```python
from build123d import *

# Parameters (mm, degrees)
SKETCH1_W       = 39
SKETCH1_H       = 39
EXTRUDE1_DEPTH  = 150
SKETCH2_W       = 36
SKETCH2_H       = 36
EXTRUDE2_DEPTH  = 112
SKETCH3_W       = 4.5
SKETCH3_H       = 120
EXTRUDE3_DEPTH  = 158.167148993
SKETCH8_W       = 36
SKETCH8_H       = 33
EXTRUDE6_DEPTH  = 2
FILLET1_R       = 1.5
SKETCH11_W      = 23.29
SKETCH11_H      = 15
EXTRUDE8_DEPTH  = 158.167148993
EXTRUDE9_DEPTH  = 1.5
SKETCH14_R      = 1.45
EXTRUDE11_DEPTH = 1.5
SKETCH15_R      = 10.365721684
EXTRUDE12_DEPTH = 158.167148993
SKETCH17_W      = 4.5
SKETCH17_H      = 1
EXTRUDE14_DEPTH = 158.167148993
SKETCH18_W      = 34.5
SKETCH18_H      = 34.16
EXTRUDE15_DEPTH = 158.167148993
SKETCH19_W      = 5
SKETCH19_H      = 10.5
EXTRUDE16_DEPTH = 10
SKETCH20_W      = 5
SKETCH20_H      = 10.5
EXTRUDE17_DEPTH = 10
SKETCH21_R      = 1.6
EXTRUDE18_DEPTH = 10
SKETCH22_R      = 1.6
EXTRUDE19_DEPTH = 10
EXTRUDE20_DEPTH = 5
SKETCH25_R      = 10
EXTRUDE21_DEPTH = 5
EXTRUDE23_DEPTH = 4
FILLET2_R       = 10
FILLET3_R       = 2


with BuildPart() as part:
    # Sketch1 → Extrude1 (new body)
    with BuildSketch(Plane(origin=(0, 0, 0), x_dir=(1, 0, 0), z_dir=(0, 1, 0))):
        with Locations((-11.707942094, -6.586638776)):
            Rectangle(SKETCH1_W, SKETCH1_H)
    extrude(amount=EXTRUDE1_DEPTH)

    # Sketch2 → Extrude2 (cut)
    with BuildSketch(Plane(origin=(0, 150, 0), x_dir=(1, 0, 0), z_dir=(0, 1, 0))):
        with Locations((-11.707942094, -6.586638776)):
            Rectangle(SKETCH2_W, SKETCH2_H)
    extrude(amount=-EXTRUDE2_DEPTH, mode=Mode.SUBTRACT)

    # Sketch3 → Extrude3 (cut, through all)
    with BuildSketch(Plane.ZY.offset(31.207942094)):
        with Locations((23.836638776, 60)):
            Rectangle(SKETCH3_W, SKETCH3_H)
    extrude(amount=-EXTRUDE3_DEPTH, mode=Mode.SUBTRACT)

    # Sketch8 → Extrude6 (cut)
    with BuildSketch(Plane(origin=(0, 38, 0), x_dir=(1, 0, 0), z_dir=(0, 1, 0))):
        with Locations((-11.707942094, -5.086638776)):
            Rectangle(SKETCH8_W, SKETCH8_H)
    extrude(amount=-EXTRUDE6_DEPTH, mode=Mode.SUBTRACT)

    # Fillet1
    fillet1_edges = [part.edges().sort_by_distance(p)[0] for p in [
        (-29.707942094, 93, -11.413361224),
        (6.292057906, 93, -11.413361224),
        (6.292057906, 135, 24.586638776),
        (-29.707942094, 135, 24.586638776),
        (6.292057906, 36, 5.086638776),
        (-29.707942094, 36, 5.086638776),
        (-11.707942094, 36, -11.413361224),
    ]]
    fillet(fillet1_edges, radius=FILLET1_R)

    # Sketch11 → Extrude8 (cut, through all)
    with BuildSketch(Plane.ZY.offset(31.207942094)):
        with BuildLine():
            Line((-3.255937041, 62.910708566), (-3.255937041, 92.357092416))
            ThreePointArc((-3.255937041, 92.357092416), (3.739612713, 99.352642171), (10.735162468, 92.357092416))
            Line((10.735162468, 92.357092416), (10.735162468, 62.910708566))
            ThreePointArc((10.735162468, 62.910708566), (3.739612713, 55.915158812), (-3.255937041, 62.910708566))
        make_face()
        with Locations((6.591638776, 142.5)):
            Rectangle(SKETCH11_W, SKETCH11_H)
    extrude(amount=-EXTRUDE8_DEPTH, mode=Mode.SUBTRACT)

    # Sketch12 → Extrude9 (cut)
    with BuildSketch(Plane(origin=(0, 0, -12.913361224), x_dir=(-1, 0, 0), z_dir=(0, 0, -1))):
        with BuildLine():
            Line((5.065703237, 62.27828297), (5.065703237, 91.808021534))
            ThreePointArc((5.065703237, 91.808021534), (11.707942094, 98.450260391), (18.350180951, 91.808021534))
            Line((18.350180951, 91.808021534), (18.350180951, 62.27828297))
            ThreePointArc((18.350180951, 62.27828297), (11.707942094, 55.636044113), (5.065703237, 62.27828297))
        make_face()
        with BuildLine():
            Line((6.527758749, 115.3801061), (6.527758749, 136.80161472))
            ThreePointArc((6.527758749, 136.80161472), (11.707942094, 141.981798065), (16.888125439, 136.80161472))
            Line((16.888125439, 136.80161472), (16.888125439, 115.3801061))
            ThreePointArc((16.888125439, 115.3801061), (11.707942094, 110.199922755), (6.527758749, 115.3801061))
        make_face()
    extrude(amount=-EXTRUDE9_DEPTH, mode=Mode.SUBTRACT)

    # Sketch14 → Extrude11 (cut)
    with BuildSketch(Plane.XY.offset(26.086638776)):
        with Locations((-5.707942094, 138.35)):
            Circle(SKETCH14_R)
        with Locations((-17.707942094, 138.35)):
            Circle(SKETCH14_R)
    extrude(amount=-EXTRUDE11_DEPTH, mode=Mode.SUBTRACT)

    # Sketch15 → Extrude12 (cut, through all)
    with BuildSketch(Plane.ZY.offset(31.207942094)):
        with Locations((3.739612713, 119.241924714)):
            Circle(SKETCH15_R)
    extrude(amount=-EXTRUDE12_DEPTH, mode=Mode.SUBTRACT)

    # Sketch17 → Extrude14 (cut, through all)
    with BuildSketch(Plane.ZY.offset(31.207942094)):
        with Locations((23.836638776, 120.5)):
            Rectangle(SKETCH17_W, SKETCH17_H)
    extrude(amount=-EXTRUDE14_DEPTH, mode=Mode.SUBTRACT)

    # Sketch18 → Extrude15 (cut, through all)
    with BuildSketch(Plane.ZY.offset(31.207942094)):
        with Locations((4.336638776, 17.08)):
            Rectangle(SKETCH18_W, SKETCH18_H)
    extrude(amount=-EXTRUDE15_DEPTH, mode=Mode.SUBTRACT)

    # Sketch19 → Extrude16 (add)
    with BuildSketch(Plane.ZY.offset(31.207942094)):
        with Locations((19.086638776, 39.41)):
            Rectangle(SKETCH19_W, SKETCH19_H)
    extrude(amount=EXTRUDE16_DEPTH)

    # Sketch20 → Extrude17 (add)
    with BuildSketch(Plane(origin=(7.792057906, 0, 0), x_dir=(0, 0, -1), z_dir=(1, 0, 0))):
        with Locations((-19.086638776, 39.41)):
            Rectangle(SKETCH20_W, SKETCH20_H)
    extrude(amount=EXTRUDE17_DEPTH)

    # Sketch21 → Extrude18 (cut)
    with BuildSketch(Plane(origin=(0, 0, 16.586638776), x_dir=(-1, 0, 0), z_dir=(0, 0, -1))):
        with Locations((-12.792057906, 39.16)):
            Circle(SKETCH21_R)
    extrude(amount=-EXTRUDE18_DEPTH, mode=Mode.SUBTRACT)

    # Sketch22 → Extrude19 (cut)
    with BuildSketch(Plane(origin=(0, 0, 16.586638776), x_dir=(-1, 0, 0), z_dir=(0, 0, -1))):
        with Locations((36.207942094, 39.16)):
            Circle(SKETCH22_R)
    extrude(amount=-EXTRUDE19_DEPTH, mode=Mode.SUBTRACT)

    # Sketch24 → Extrude20 (add)
    with BuildSketch(Plane(origin=(0, 0, 16.586638776), x_dir=(-1, 0, 0), z_dir=(0, 0, -1))):
        Polygon((-17.792057906, 44.66), (-7.792057906, 44.66), (-7.792057906, 54.66), align=None)
        Polygon((41.207942094, 44.66), (31.207942094, 44.66), (31.207942094, 54.66), align=None)
    extrude(amount=-EXTRUDE20_DEPTH)

    # Sketch25 → Extrude21 (cut)
    with BuildSketch(Plane(origin=(0, 34.16, 0), x_dir=(-1, 0, 0), z_dir=(0, -1, 0))):
        with Locations(Location((11.707942094, -2.086638776, 0), (0, 0, 90))):
            Circle(SKETCH25_R)
    extrude(amount=-EXTRUDE21_DEPTH, mode=Mode.SUBTRACT)

    # Sketch31 → Extrude23 (add)
    with BuildSketch(Plane(origin=(0, 43.16, 0), x_dir=(-1, 0, 0), z_dir=(0, -1, 0))):
        Polygon((-12.792057906, -16.586638776), (-7.792057906, -16.586638776), (-7.792057906, -10.735162468), align=None)
        Polygon((36.207942094, -16.586638776), (31.207942094, -16.586638776), (31.207942094, -11.586638776), align=None)
    extrude(amount=-EXTRUDE23_DEPTH)

    # Fillet2
    fillet2_edges = [part.edges().sort_by_distance(p)[0] for p in [
        (7.792057906, 54.66, 19.086638776),
        (-31.207942094, 54.66, 19.086638776),
    ]]
    fillet(fillet2_edges, radius=FILLET2_R)

    # Fillet3
    fillet3_edges = [part.edges().sort_by_distance(p)[0] for p in [
        (7.792057906, 45.16, 10.735162468),
        (12.792057906, 45.16, 16.586638776),
        (-31.207942094, 45.16, 11.586638776),
        (-36.207942094, 45.16, 16.586638776),
    ]]
    fillet(fillet3_edges, radius=FILLET3_R)


solid = part.part
```
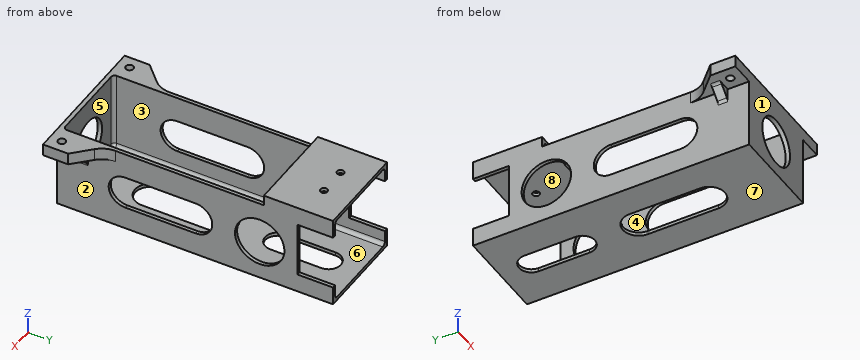
Source: CAD feature listing. Evaluate the final solid. Frame: model axes, mm. Face numbers are marked on the shaded views. A direction names the side the tool comes from. Coordinates: 2 decimals unless noted, no trailing zeros. Order: outer loops, then holes, each group sorted by start corner. A loop starts at its lowest first (then second) coordinate and runs counter-clockwise, first axis right, second up. Notation, with made-up numbers: (-24.5, 14) - (-8.5, 14) arc R15 cw to (-8.5, 39) - close; hole circle Ø4 at (36.5, 32). An arc over 180 degrees is marked (long way). One line per item, written item: value.
1) Cut plane B-B on z = 3. State how many separate pieces and enclosed holes the cut face has, plus the area to 3 significant figures.
Computed values:
separate pieces: 6
enclosed holes: 0
area: 141 mm^2
2) Ray query, line 1 (X direction, y = 138.35, z = 25); line 2 (X direction, y = 39, z = 20); line 3 (Z direction, x = 7, y = 81.5). Return the intervals inside material, ascending. Write a range as [from, to].
Computed values:
line 1: x = [-31.21, -19.16], [-16.26, -7.16], [-4.26, 7.79]
line 2: x = [-41.21, -37.8], [-34.62, -29.71], [6.29, 11.2], [14.38, 17.79]
line 3: z = [-12.91, -3.26], [10.74, 21.59]
3) Cut plane A-A on y = 39.16. Output: boundary loops of the cut face in (x, z).
Computed values:
outline: (-41.21, 16.59) - (-37.81, 16.59) - (-37.81, 21.59) - (-41.21, 21.59) - close; (-34.61, 16.59) - (-31.21, 16.59) - (-31.21, -12.91) - (7.79, -12.91) - (7.79, 16.59) - (11.19, 16.59) - (11.19, 21.59) - (6.29, 21.59) - (6.29, -9.91) arc R1.5 cw to (4.79, -11.41) - (-28.21, -11.41) arc R1.5 cw to (-29.71, -9.91) - (-29.71, 21.59) - (-34.61, 21.59) - close; (14.39, 16.59) - (17.79, 16.59) - (17.79, 21.59) - (14.39, 21.59) - close
4) Cut plane D-D on x = -20.5. Output: boundary loops of the cut face in (y, z).
Computed values:
outline: (34.16, -12.91) - (150, -12.91) - (150, -11.41) - (37.5, -11.41) arc R1.5 cw to (36, -9.91) - (36, -2.68) - (34.16, -2.68) - close; (34.16, 6.85) - (36, 6.85) - (36, 21.59) - (34.16, 21.59) - close; (121, 24.59) - (150, 24.59) - (150, 26.09) - (121, 26.09) - close
5) Reachability of the marked faces 5, 6, 7 and 8 from +Z, -Z, +X, -X, +Y, -Y: full face, straight path, thin tool, end or side. Return the list, or none.
Computed values:
face 5: +Z, +Y
face 6: +Y
face 7: -Z, +X, -X, +Y, -Y
face 8: +Y, -Y
6) Mould query, pull axis X, two halves, no side actions, for the marked faces 1, 2, 3 and 4. Classes: released by +X, released by -X, zero draft, split by the parting line, or undercut.
Computed values:
face 1: zero draft
face 2: released by +X
face 3: undercut
face 4: undercut
7) Contact query for flat-ended pins moving along their axis: pin 1 (2 mm diameter, centred on y = 61.5, z = -7, fed in from +X); pin 2 (4.5 mm diameter, centred on x = 11, z = 13, fed in from -Y); pin 3 (6 mm diameter, centred on y = 74.5, z = -6, fed in from -X); pin 4 (3.5 mm diameter, centred on x = -17.71, y = 138.35, fed in from +Z). Output: stop coordinate, or through.
Computed values:
pin 1: stops at x = 7.79
pin 2: stops at y = 43.16
pin 3: stops at x = -31.21
pin 4: stops at z = 26.09
8) Cut plane C-C on y = 74.5. Output: boundary loops of the cut face in (x, z).
Computed values:
outline: (-31.21, -12.91) - (-18.35, -12.91) - (-18.35, -11.41) - (-28.21, -11.41) arc R1.5 cw to (-29.71, -9.91) - (-29.71, -3.26) - (-31.21, -3.26) - close; (-31.21, 10.74) - (-29.71, 10.74) - (-29.71, 21.59) - (-31.21, 21.59) - close; (-5.07, -12.91) - (7.79, -12.91) - (7.79, -3.26) - (6.29, -3.26) - (6.29, -9.91) arc R1.5 cw to (4.79, -11.41) - (-5.07, -11.41) - close; (6.29, 10.74) - (7.79, 10.74) - (7.79, 21.59) - (6.29, 21.59) - close
